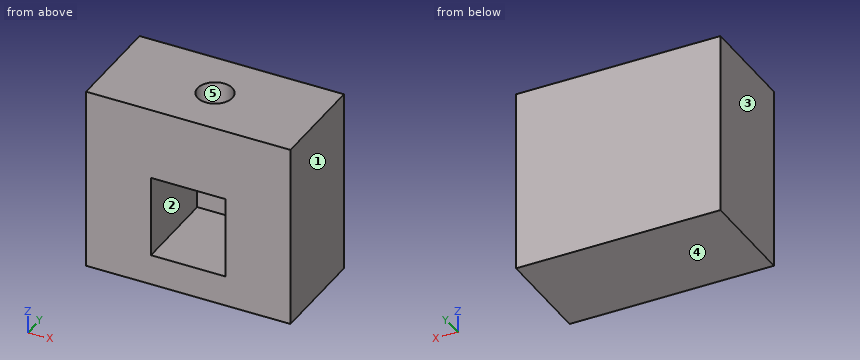
from build123d import *

# Parameters (mm, degrees)
SKETCH1_W           = 20
SKETCH1_H           = 18
BOSS_EXTRUDE1_DEPTH = 10
SKETCH2_R           = 1.705
CUT_EXTRUDE1_DEPTH  = 15
SKETCH3_W           = 7.3
SKETCH3_H           = 8.65
CUT_EXTRUDE2_DEPTH  = 8


with BuildPart() as part:
    # Sketch1 → Boss-Extrude1 (new body)
    with BuildSketch(Plane(origin=(0, 0, 0), x_dir=(1, 0, 0), z_dir=(0, 1, 0))):
        with Locations((-18, -29)):
            Rectangle(SKETCH1_W, SKETCH1_H)
    extrude(amount=BOSS_EXTRUDE1_DEPTH)

    # Sketch2 → Cut-Extrude1 (cut)
    with BuildSketch(Plane.XY.offset(38)):
        with Locations((-18, 5)):
            Circle(SKETCH2_R)
    extrude(amount=-CUT_EXTRUDE1_DEPTH, mode=Mode.SUBTRACT)

    # Sketch3 → Cut-Extrude2 (cut)
    with BuildSketch(Plane.XY.offset(23)):
        with Locations((-18, 4.325)):
            Rectangle(SKETCH3_W, SKETCH3_H)
    extrude(amount=CUT_EXTRUDE2_DEPTH, mode=Mode.SUBTRACT)


solid = part.part
Check sheet for the modelled part. Datum: model origin and axes. Units: mm. Face numbers are marked on the shaded views. A direction names the side the tool comes from. Give positions to 0.01 mm unless a question says otherwise; leave off trailing zeros. Loops run counter-clockwise (first coordinate to the right, second up) from the corner with the lowest first, then second, coordinate; pieces in that order, holes last. Notation, with made-up numbers: M 51,72.25 L 103,72.25 A11 ccw 103,85.25 Z; hole C -28.5,81.5 d5. An arc over 180 degrees is marked long. Answer as a JSON object with one key per item and string values. Group by question number.
Q1. Cross-section at D-D on y = 5. Record the cut outline in (x, z) (3 decimals), then the cut area to 3 significant figures.
Q2. Release check for a two-part mould opening along X. For the marked faces 3, 4 and 5 record: released by +X, released by -X, zero draft, split by the parting line, or undercut.
Q3. Cross-section at B-B on y = 7.5. Record the cut outline in (x, z), then the cut area to 3 significant figures.
Q4. Access from +Z, -Z, +X, -X, +Y, -Y to the whole of each face (thin tool, end or side, straight path). Record for the marked faces 1 and 2.
Q5. Cross-section at A-A on x = -18. Record the cut outline in (y, z) (3 decimals), then the cut area to 3 significant figures.
Q6. Cross-section at C-C on z = 31.5. Record the cut outline in (x, y) (3 decimals).
Q7. Go/stop test with a flat-tipped pin: P1, Ø3.5, axis at x = -17, y = 6, coming from the +Z side. Record where the tip stops, or that it passes through.
Q8. Material ranges on line 1 along X through (y, z) = (7.5, 23.25); line 2 along Z through (x, y) = (-20.5, 7.75); line 3 along Y through (x, z) = (-18, 35) (3 decimals), recorded low to high. Write a range as [from, to].
Evaluation:
{
 "1": {"outline": "M -28,20 L -8,20 L -8,38 L -16.295,38 L -16.295,31 L -14.35,31 L -14.35,23 L -21.65,23 L -21.65,31 L -19.705,31 L -19.705,38 L -28,38 Z", "area": "278 mm2"},
 "2": {"face 3": "released by -X", "face 4": "zero draft", "face 5": "undercut"},
 "3": {"outline": "M -28,20 L -8,20 L -8,38 L -28,38 Z; hole M -21.65,23 L -14.35,23 L -14.35,31 L -21.65,31 Z", "area": "302 mm2"},
 "4": {"face 1": "+Z, -Z, +X, +Y, -Y", "face 2": "-Y"},
 "5": {"outline": "M 0,20 L 10,20 L 10,38 L 6.705,38 L 6.705,31 L 8.65,31 L 8.65,23 L 0,23 Z; M 0,31 L 3.295,31 L 3.295,38 L 0,38 Z", "area": "86.9 mm2"},
 "6": {"outline": "M -28,0 L -8,0 L -8,10 L -28,10 Z; hole C -18,5 d3.41"},
 "7": {"P1": "stops at z = 38"},
 "8": {"line 1": "x = [-28, -21.65], [-14.35, -8]", "line 2": "z = [20, 23], [31, 38]", "line 3": "y = [0, 3.295], [6.705, 10]"}
}
